The figure shows three views and two pictorial views of one solid part (mm, origin at its lowest corner). Answer the questions. A direction names the side the tool comes from. Give positions to 0.01 mm unless a question says otherwise; leave off trailing zeros. Write each loop counter-clockwise with the first axis right and the second up, starting at its lowest first coordinate (ties: lowest second). Pieces come first, ordered by that corner, then holes. Notation, with made-up numbers: (21.25, 22) -> (44.25, 22) arc R14 ccw to (44.25, 37) -> close; hole circle Ø11 at (34.25, 10.5). An arc over 180 degrees is marked (long way). Answer as CSV lines item,"result". Start each with the question number.
1. The part is cut by section C-C, the plane z = 72. Determine the outline of the cut face in (x, y) (1 decimal).
2. Find the intervals of material crossed by line 1 (X direction, y = 52, z = 98.5); line 2 (Z direction, x = 298.5, y = 54.5); line 3 (X direction, y = 36, z = 76) (1 decimal), in increasing order.
3. The part is cut by section A-A, the plane z = 98. Determine the outline of the cut face in (x, y).
4. The part is cut by section D-D, the plane x = 191.5. Determine the outline of the cut face in (y, z) (1 decimal).
5. Given pin 1 (5.5 mm diameter, centred on x = 9.74, y = 47.62, fed in from -Z); pin 2 (8.5 mm diameter, centred on x = 9.74, y = 15.88, fed in from +Z); pin 3 (1.5 mm diameter, centred on x = 211.5, y = 27, fed in from -Z); pin 4 (12 mm diameter, centred on y = 53.5, z = 76, fed in from +X), each flat-ended and moving along its own axis, determine where each tip first touches the part or whether it passes through.
6. A tool of negligible diameter and unlimited length cuts with its end or side. For the marked faces 1, 2 and 3, from which of +Z, -Z, +X, -X, +Y, -Y can it reach the whole face along a straight path? Write none if from no direction.
7. The part is cut by section B-B, the plane y = 5.5. Determine the outline of the cut face in (x, z), and give its area (3 significant figures).
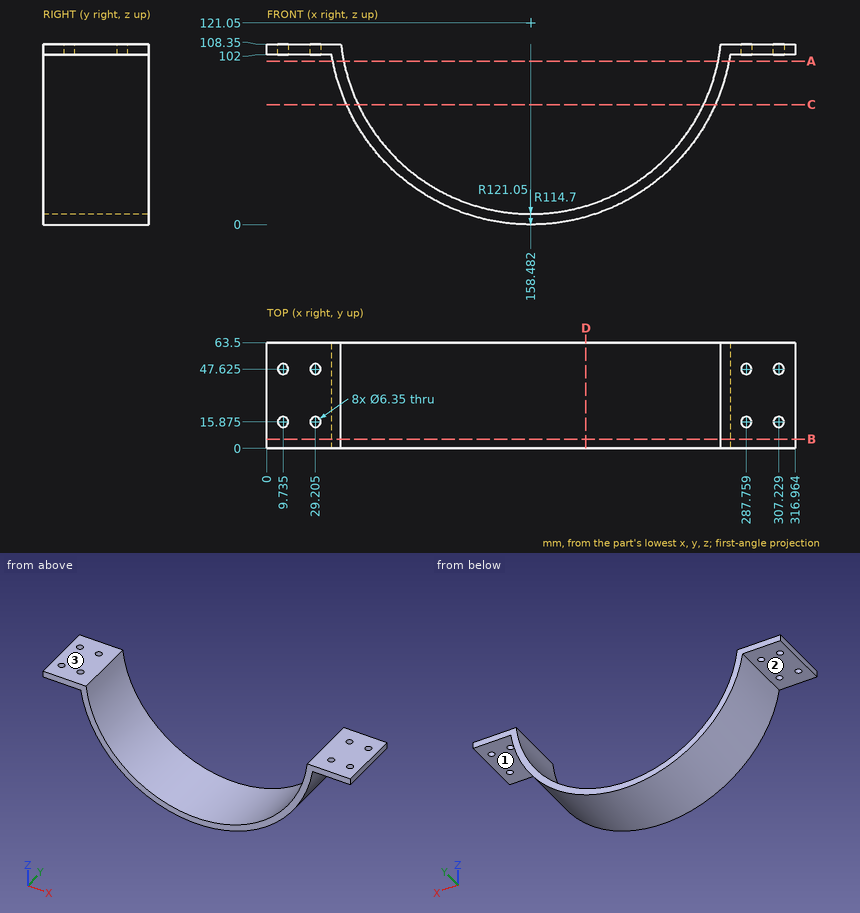
Results found:
1,outline,"(47.8, 0) -> (54.8, 0) -> (54.8, 63.5) -> (47.8, 63.5) -> close; (262.2, 0) -> (269.1, 0) -> (269.1, 63.5) -> (262.2, 63.5) -> close"
2,line 1,"x = 39.55 to 46.02, 270.94 to 277.41"
2,line 2,"z = 102 to 108.35"
2,line 3,"x = 46.1 to 53, 264 to 270.8"
3,outline,"(39.65, 0) -> (46.12, 0) -> (46.12, 63.5) -> (39.65, 63.5) -> close; (270.84, 0) -> (277.32, 0) -> (277.32, 63.5) -> (270.84, 63.5) -> close"
4,outline,"(0, 4.6) -> (63.5, 4.6) -> (63.5, 11.2) -> (0, 11.2) -> close"
5,pin 1,"passes through"
5,pin 2,"stops at z = 108.35"
5,pin 3,"stops at z = 11.87"
5,pin 4,"stops at x = 273.06"
6,face 1,"-Z, +X, +Y, -Y"
6,face 2,"-Z, -X, +Y, -Y"
6,face 3,"+Z, +X, -X, +Y, -Y"
7,outline,"(0, 102) -> (38.94, 102) arc R121.05 ccw to (278.02, 102) -> (316.96, 102) -> (316.96, 108.35) -> (272.48, 108.35) arc R114.7 cw to (44.49, 108.35) -> (0, 108.35) -> close"
7,area,"2,680 mm²"
